from build123d import *

# Parameters (mm, degrees)
SKETCH1_R           = 7.5
BOSS_EXTRUDE1_DEPTH = 10
BOSS_EXTRUDE1_TAPER = 10
SKETCH2_R           = 5.625
CUT_EXTRUDE1_DEPTH  = 2.25
FILLET1_R           = 2


# Read off the part's stored shape, not the designer's step: Shell2
with BuildPart() as part:
    # Sketch1 → Boss-Extrude1 (new body)
    with BuildSketch(Plane(origin=(0, 0, 0), x_dir=(1, 0, 0), z_dir=(0, 1, 0))):
        Circle(SKETCH1_R)
    extrude(amount=BOSS_EXTRUDE1_DEPTH, taper=BOSS_EXTRUDE1_TAPER)

    # Sketch2 → Cut-Extrude1 (cut)
    with BuildSketch(Plane.XZ):
        with Locations(Location((0, 0, 0), (0, 0, 270))):
            Circle(SKETCH2_R)
    extrude(amount=-CUT_EXTRUDE1_DEPTH, mode=Mode.SUBTRACT)

    # Fillet1
    fillet1_edges = [part.edges().sort_by_distance(p)[0] for p in [
        (-5.736730193, 10, 0),
    ]]
    fillet(fillet1_edges, radius=FILLET1_R)

    # Shell2 outline → Shell2 (revolve, cut)
    with BuildSketch(Plane.XY):
        with BuildLine():
            Line((5.580124376, 2.25), (4.550934807, 8.086824089))
            ThreePointArc((4.550934807, 8.086824089), (4.379924736, 8.383022222), (4.058530931, 8.5))
            Line((4.058530931, 8.5), (0, 8.5))
            Line((0, 8.5), (0, 2.25))
            Line((0, 2.25), (5.580124376, 2.25))
        make_face()
    revolve(axis=Axis((0, 0, 0), (0, 1, 0)), mode=Mode.SUBTRACT)


solid = part.part
Here's how the part is built. I have some questions about the finished solid (model axes, mm). A direction names the side the tool comes from. Coordinates: 2 decimals unless noted, no trailing zeros. Loops run counter-clockwise (first coordinate to the right, second up) from the corner with the lowest first, then second, coordinate; pieces in that order, holes last.
1. Imagine slicing it at A-A, the plane x = 0. Please give me the cut outline in (y, z) (3 decimals), and give its area (3 significant figures).
2. I need wall thicknesses on L1, parallel to Y at x = 0.5, z = -3.75; L2, parallel to X at y = 1.25, z = 4.75; L3, parallel to X at y = 0.9, z = 0 (3 decimals). Which ranges of each line are inside material? Lowest first, please.
3. If we mould it in two halves opening along X, with no side actions, what happens to faces 1 (the flat face through (1, 0, -6)), 2 (the conical face through (3.54, 5.16, -5.56)), 3 (the cylindrical face through (-2.15, 1.11, -5.2))? For each: pulls with the +X half, pulls with the -X half, needs draft (parallel to the pull), parting line crosses it, or undercut.
4. For P1, Ø1.5, axis at y = 3, z = 1.5, coming from the -X side; P2, Ø1, axis at x = 3, y = 6.5, coming from the +Z side; P3, Ø5, axis at x = 2, y = 5, coming from the -Z side, each with a flat end and sliding along its axis, tell me the tip position at first contact or that it passes through.
5. For faces 4 (the flat face through (0, 10, 0)), 5 (the flat face through (0, 8.5, 0)), which set-ups out of +Z, -Z, +X, -X, +Y, -Y let a thin tool reach every point of the face, with its end or its side?
6. Imagine slicing it at B-B, the plane y = 4. Please give me the cut outline in (x, z).
Taken from the geometry:
1. outline: (0, -7.5) - (8.347, -6.028) arc R2 ccw to (10, -4.059) - (10, 4.059) arc R2 ccw to (8.347, 6.028) - (0, 7.5) - (0, 5.625) - (2.25, 5.625) - (2.25, 5.58) - (8.087, 4.551) arc R0.5 cw to (8.5, 4.059) - (8.5, -4.059) arc R0.5 cw to (8.087, -4.551) - (2.25, -5.58) - (2.25, -5.625) - (0, -5.625) - close
1. area: 43.1 mm2
2. L1: y = 8.5 to 10
2. L2: x = -5.52 to -3.01, 3.01 to 5.52
2. L3: x = -7.341 to -5.625, 5.625 to 7.341
3. face 1: needs draft
3. face 2: parting line crosses it
3. face 3: undercut
4. P1: stops at x = -7
4. P2: stops at z = 5.86
4. P3: stops at z = -6.96
5. face 4: +Z, -Z, +X, -X, +Y
5. face 5: -Y
6. outline: circle Ø13.59 at (0, 0); hole circle Ø10.54 at (0, 0)
